Model file for the job. Use its own axes, mm. A direction names the side the tool comes from. Round coordinates to 2 decimals unless told otherwise and drop trailing zeros. Loops run counter-clockwise (first coordinate to the right, second up) from the corner with the lowest first, then second, coordinate; pieces in that order, holes last. Notation, with made-up numbers: (33, 39) - (41, 39) arc R26 cw to (41, 62) - close; hole circle Ø3 at (12, 2). An arc over 180 degrees is marked (long way). Use one line per item in the form item = value.
from build123d import *

# Parameters (mm, degrees)
SKETCH1_R           = 70
BOSS_EXTRUDE1_DEPTH = 30
SHELL1_T            = -2
SKETCH2_R           = 33
SKETCH2_R_2         = 29
EXTRUDE_THIN1_DEPTH = 5
SKETCH3_R           = 33
SKETCH3_R_2         = 30
CUT_EXTRUDE1_DEPTH  = 5
SKETCH4_R           = 29
CUT_EXTRUDE2_DEPTH  = 2
SKETCH5_R           = 3
CUT_EXTRUDE3_DEPTH  = 5


with BuildPart() as part:
    # Sketch1 → Boss-Extrude1 (new body)
    with BuildSketch(Plane(origin=(0, 0, 0), x_dir=(1, 0, 0), z_dir=(0, 1, 0))):
        with Locations(Location((0, 0, 0), (0, 0, 270))):
            Circle(SKETCH1_R)
    extrude(amount=BOSS_EXTRUDE1_DEPTH)

    # Shell1
    shell1_openings = [part.faces().sort_by_distance(p)[0] for p in [
        (0, 30, 0),
    ]]
    offset(amount=SHELL1_T, openings=shell1_openings, kind=Kind.INTERSECTION)

    # Sketch2 → Extrude-Thin1 (add)
    with BuildSketch(Plane(origin=(0, 2, 0), x_dir=(1, 0, 0), z_dir=(0, 1, 0))):
        with Locations((34.921312676, 0)):
            Circle(SKETCH2_R)
        with Locations((34.921312676, 0)):
            Circle(SKETCH2_R_2, mode=Mode.SUBTRACT)
    extrude(amount=EXTRUDE_THIN1_DEPTH)

    # Sketch3 → Cut-Extrude1 (cut)
    with BuildSketch(Plane(origin=(0, 7, 0), x_dir=(1, 0, 0), z_dir=(0, 1, 0))):
        with Locations((34.921312676, 0)):
            Circle(SKETCH3_R)
        with Locations(Location((34.921312676, 0, 0), (0, 0, 270))):
            Circle(SKETCH3_R_2, mode=Mode.SUBTRACT)
    extrude(amount=-CUT_EXTRUDE1_DEPTH, mode=Mode.SUBTRACT)

    # Sketch4 → Cut-Extrude2 (cut)
    with BuildSketch(Plane(origin=(0, 2, 0), x_dir=(1, 0, 0), z_dir=(0, 1, 0))):
        with Locations(Location((34.921312676, 0, 0), (0, 0, 270))):
            Circle(SKETCH4_R)
    extrude(amount=-CUT_EXTRUDE2_DEPTH, mode=Mode.SUBTRACT)

    # Sketch5 → Cut-Extrude3 (cut, symmetric)
    with BuildSketch(Plane(origin=(0, 2, 0), x_dir=(1, 0, 0), z_dir=(0, 1, 0))):
        with Locations(Location((-60, 0, 0), (0, 0, 270))):
            Circle(SKETCH5_R)
    extrude(amount=CUT_EXTRUDE3_DEPTH, both=True, mode=Mode.SUBTRACT)


solid = part.part
1. Cut at D-D, the plane x = 0. Give the cut face in (y, z).
Geometry check:
outline = (0, -70) - (30, -70) - (30, -68) - (2, -68) - (2, 68) - (30, 68) - (30, 70) - (0, 70) - close
2. Pull direction Z, two halves, no side cores. Call faces 3 (the flat face through (68, 30, -11)), 4 (the cylindrical face through (-57, 1, 0)), 5 (the cylindrical face through (-42.594, 14.79, -55.55)): +Z half, -Z half, draft (parallel to the pull), parting line (faces both ways), or undercut.
Geometry check:
face_3 = draft
face_4 = undercut
face_5 = parting line
3. Flat gauge pins, fed straight in: pin 1 (5 mm diameter, centred on y = 14.5, z = -38.5, fed in from +X); pin 2 (1 mm diameter, centred on y = 11.5, z = -27, fed in from +X); pin 3 (8 mm diameter, centred on x = -31, z = 55, fed in from +Y); pin 4 (5.5 mm diameter, centred on x = -60, z = 0, fed in from -Y). Where does each tip first touch, or does it go through?
Geometry check:
pin_1 = 60.03
pin_2 = 64.79
pin_3 = 2
pin_4 = through
4. Cut at B-B, the plane x = -60. Give the cut face in (y, z), plus the area to 3 significant figures.
Geometry check:
outline = (0, -36.06) - (30, -36.06) - (30, -32) - (2, -32) - (2, -3) - (0, -3) - close; (0, 3) - (2, 3) - (2, 32) - (30, 32) - (30, 36.06) - (0, 36.06) - close
area = 359 mm^2
5. Cut at C-C, the plane z = -24. Give the cut face in (x, y).
Geometry check:
outline = (-65.76, 0) - (18.64, 0) - (18.64, 7) - (16.92, 7) - (16.92, 2) - (-63.62, 2) - (-63.62, 30) - (-65.76, 30) - close; (51.2, 0) - (65.76, 0) - (65.76, 30) - (63.62, 30) - (63.62, 2) - (52.92, 2) - (52.92, 7) - (51.2, 7) - close
6. Tool access for faces 1 (the flat face through (-14, 2, -1)), 2 (the flat face through (1, 0, -1)): list every direction of +Z, -Z, +X, -X, +Y, -Y with a clear straight run to the whole face (end or side of a thin tool).
Geometry check:
face_1 = +Y
face_2 = +Z, -Z, +X, -X, -Y
7. Wall check: probe 1 along X at (y, z) = (1.25, 0); probe 2 along Z at (x, y) = (33.5, 4.25); probe 3 along Y at (x, z) = (-11, 61.5). Give the ranges that are in metal, low to high.
Geometry check:
probe_1 = -70 to -63, -57 to 5.92, 63.92 to 70
probe_2 = -61.46 to -59.18, -29.97 to -28.97, 28.97 to 29.97, 59.18 to 61.46
probe_3 = 0 to 2
8. Cut at A-A, the plane z = 0. Give the cut face in (x, y), plus the area to 3 significant figures.
Geometry check:
outline = (-70, 0) - (-63, 0) - (-63, 2) - (-68, 2) - (-68, 30) - (-70, 30) - close; (-57, 0) - (5.92, 0) - (5.92, 7) - (4.92, 7) - (4.92, 2) - (-57, 2) - close; (63.92, 0) - (70, 0) - (70, 30) - (68, 30) - (68, 2) - (64.92, 2) - (64.92, 7) - (63.92, 7) - close
area = 274 mm^2
